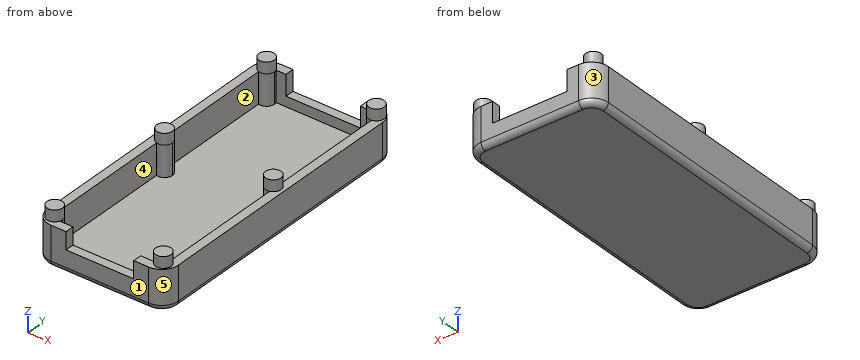
```python
from build123d import *

# Parameters (mm, degrees)
SKETCH1_W                = 23.6
SKETCH1_H                = 53
BOSS_EXTRUDE2_DEPTH      = 7.1
SHELL1_T                 = -1.6
FILLET2_R                = 3
SKETCH7_W                = 12.2
SKETCH7_H                = 1.6
CUT_EXTRUDE1_DEPTH       = 3.1
SKETCH8_W                = 13.4
SKETCH8_H                = 1.6
CUT_EXTRUDE2_DEPTH       = 3.7
FILLET3_R                = 1
SKETCH10_R               = 1.4
BOSS_EXTRUDE4_DEPTH      = 2
BOSS_EXTRUDE4_DEPTH_BACK = 6.5


with BuildPart() as part:
    # Sketch1 → Boss-Extrude2 (new body)
    with BuildSketch(Plane.XY):
        with Locations((-28.818351302, -28.026390465)):
            Rectangle(SKETCH1_W, SKETCH1_H)
    extrude(amount=BOSS_EXTRUDE2_DEPTH)

    # Shell1
    shell1_openings = [part.faces().sort_by_distance(p)[0] for p in [
        (-28.818351302, -28.026390465, 7.1),
    ]]
    offset(amount=SHELL1_T, openings=shell1_openings, kind=Kind.INTERSECTION)

    # Fillet2
    fillet2_edges = [part.edges().sort_by_distance(p)[0] for p in [
        (-40.618351302, -1.526390465, 3.55),
        (-17.018351302, -1.526390465, 3.55),
        (-17.018351302, -54.526390465, 3.55),
        (-40.618351302, -54.526390465, 3.55),
    ]]
    fillet(fillet2_edges, radius=FILLET2_R)

    # Sketch7 → Cut-Extrude1 (cut)
    with BuildSketch(Plane.XY.offset(7.1)):
        with Locations((-28.818351302, -53.726390465)):
            Rectangle(SKETCH7_W, SKETCH7_H)
    extrude(amount=-CUT_EXTRUDE1_DEPTH, mode=Mode.SUBTRACT)

    # Sketch8 → Cut-Extrude2 (cut)
    with BuildSketch(Plane.XY.offset(7.1)):
        with Locations((-28.818351302, -2.326390465)):
            Rectangle(SKETCH8_W, SKETCH8_H)
    extrude(amount=-CUT_EXTRUDE2_DEPTH, mode=Mode.SUBTRACT)

    # Fillet3
    fillet3_edges = [part.edges().sort_by_distance(p)[0] for p in [
        (-28.818351302, -1.526390465, 0),
        (-40.618351302, -28.026390465, 0),
        (-17.018351302, -28.026390465, 0),
        (-28.818351302, -54.526390465, 0),
        (-39.739671646, -2.405070122, 0),
        (-39.739671646, -53.647710809, 0),
        (-17.897030959, -53.647710809, 0),
        (-17.897030959, -2.405070122, 0),
    ]]
    fillet(fillet3_edges, radius=FILLET3_R)

    # Sketch10 → Boss-Extrude4 (add, two sides)
    with BuildSketch(Plane.XY.offset(7.1)) as boss_extrude4_sk:
        with Locations((-38.618351302, -52.426390465)):
            Circle(SKETCH10_R)
        with Locations((-19.018351302, -52.426390465)):
            Circle(SKETCH10_R)
        with Locations((-38.618351302, -27.126390465)):
            Circle(SKETCH10_R)
        with Locations((-19.018351302, -27.126390465)):
            Circle(SKETCH10_R)
        with Locations((-18.818351302, -3.626390465)):
            Circle(SKETCH10_R)
        with Locations((-38.618351302, -3.626390465)):
            Circle(SKETCH10_R)
    extrude(amount=BOSS_EXTRUDE4_DEPTH)
    extrude(boss_extrude4_sk.sketch, amount=-BOSS_EXTRUDE4_DEPTH_BACK)


solid = part.part
```
The model under review builds one solid part; all positions refer to its coordinate system, in mm. Face numbers are marked on the shaded views. A direction names the side the tool comes from. Round coordinates to 2 decimals unless told otherwise and drop trailing zeros. Write each loop counter-clockwise with the first axis right and the second up, starting at its lowest first coordinate (ties: lowest second). Pieces come first, ordered by that corner, then holes. Notation, with made-up numbers: (27, 32.5) - (51, 32.5) arc R9 cw to (51, 43.5) - close; hole circle Ø3 at (47, 4). An arc over 180 degrees is marked (long way). Answer as CSV lines item,"result". Start each with the question number.
(1) We need section A-A on z = 6.25. State the section outline as (x, y) points, plus the area to 3 significant figures.
(2) We need section C-C on y = -15. State the section outline as (x, z) points, plus the area to 3 significant figures.
(3) For pin 1 Ø0.8 at (y, z) = (-2.5, 5) entering from +X; pin 2 Ø0.8 at (y, z) = (-2.5, 5.5) entering from -X; pin 3 Ø5 at (x, y) = (-26.5, -47) entering from +Z; pin 4 Ø6.5 at (x, y) = (-37, -25.5) entering from +Z, all flat-tipped, find the tip position at first contact; note any pin that passes through.
(4) Draft analysis for pull direction Y (two halves, no side actions). For the marked faces 3, 4 and 5, state which applies: pulls with the +Y half, pulls with the -Y half, needs draft (parallel to the pull), parting line crosses it, or undercut.
(5) We need section B-B on x = -33. State the section outline as (y, z) points.
(6) For the marked faces 1 and 2, list the 3-axis set-ups (+Z, -Z, +X, -X, +Y, -Y) from which the entire face can be reached by the end or side of a thin tool; tool diameter is ignored.
(7) To check wall thickness, follow line 1 (X direction, y = -44.5, z = 2.75); line 2 (Y direction, x = -38.25, z = 5.5); line 3 (Y direction, x = -20, z = 4.75). State the ranges of each line that lie inside material, in increasing order.
Worked answers:
1,outline,"(-40.62, -51.53) arc R3 ccw to (-37.62, -54.53) - (-34.92, -54.53) - (-34.92, -52.93) - (-37.31, -52.93) arc R1.4 ccw to (-39.02, -51.08) - (-39.02, -28.47) arc R1.4 ccw (long way) to (-39.02, -25.78) - (-39.02, -4.97) arc R1.4 ccw to (-37.31, -3.13) - (-35.52, -3.13) - (-35.52, -1.53) - (-37.62, -1.53) arc R3 ccw to (-40.62, -4.53) - close; (-22.72, -54.53) - (-20.02, -54.53) arc R3 ccw to (-17.02, -51.53) - (-17.02, -4.53) arc R3 ccw to (-20.02, -1.53) - (-22.12, -1.53) - (-22.12, -3.13) - (-20.13, -3.13) arc R1.4 ccw to (-18.62, -5.01) - (-18.62, -25.78) arc R1.4 ccw (long way) to (-18.62, -28.47) - (-18.62, -51.08) arc R1.4 ccw to (-20.33, -52.93) - (-22.72, -52.93) - close"
1,area,"206 mm²"
2,outline,"(-40.62, 1) arc R1 ccw to (-39.62, 0) - (-18.02, 0) arc R1 ccw to (-17.02, 1) - (-17.02, 7.1) - (-18.62, 7.1) - (-18.62, 1.6) - (-39.02, 1.6) - (-39.02, 7.1) - (-40.62, 7.1) - close"
2,area,"54.9 mm²"
3,pin 1,"x = -17.5"
3,pin 2,"x = -40.14"
3,pin 3,"z = 1.6"
3,pin 4,"z = 9.1"
4,face 3,"pulls with the +Y half"
4,face 4,"undercut"
4,face 5,"pulls with the -Y half"
5,outline,"(-54.53, 1) arc R1 ccw to (-53.53, 0) - (-2.53, 0) arc R1 ccw to (-1.53, 1) - (-1.53, 3.4) - (-3.13, 3.4) - (-3.13, 1.6) - (-52.93, 1.6) - (-52.93, 4) - (-54.53, 4) - close"
6,face 1,"+Z, -Z, +X, -X, -Y"
6,face 2,"+Z"
7,line 1,"-40.62 to -39.02, -18.62 to -17.02"
7,line 2,"-54.46 to -51.08, -28.48 to -25.78, -4.98 to -1.59"
7,line 3,"-54.53 to -51.43, -28.12 to -26.13, -4.38 to -1.53"
